Source: CAD feature listing. Evaluate the final solid. Frame: model axes, mm. A direction names the side the tool comes from. Round coordinates to 2 decimals unless told otherwise and drop trailing zeros. Loops run counter-clockwise (first coordinate to the right, second up) from the corner with the lowest first, then second, coordinate; pieces in that order, holes last. Notation, with made-up numbers: (6, 3.25) -> (10, 3.25) arc R21 ccw to (10, 42.25) -> close; hole circle Ø4 at (-6, -5.5). An arc over 180 degrees is marked (long way). Put each result on its own line as item: value. Start each with the question number.
1. Cut plane A-A (y = 0). Return the cut outline in (x, z), then the cut area to 3 significant figures.
2. Cut plane D-D (y = 7.25). Return the cut outline in (x, z).
3. Cut plane B-B (z = 1). Return the cut outline in (x, y).
4. Cut plane C-C (x = 0). Return the cut outline in (y, z), then the cut area to 3 significant figures.
5. Set-up query: faces 1 (the flat face through (-14.345, 6.755, 2.465)), 2 (the flat face through (-2, 6, 5)). Return all of +Z, -Z, +X, -X, +Y, -Y with unobstructed straight access to the full face (end or side cutting, diameter ignored); none if empty.
6. Material intervals for L1, parallel to Y at x = 0, z = 6.2; L2, parallel to Z at x = -26, y = -1.5; L3, parallel to Y at x = 0, z = 2.7, sorted ascending.
7. Draft query along X for faces 3 (the flat face through (-14.015, -6.836, 2.465)), 4 (the cylindrical face through (-6, 0, 6)), 5 (the cylindrical face through (-1.73, -7.81, 2.46)), 6 (the flat face through (0, -7, 7)). Return one class per face: pulls with the +X half, pulls with the -X half, needs draft (parallel to the pull), parting line crosses it, or undercut.
8. Contact query for flat-ended pins moving along their axis: pin 1 (3 mm diameter, centred on x = -21.5, z = 5.5, fed in from -Y); pin 2 (1.5 mm diameter, centred on x = -20.5, y = 0, fed in from -Z); pin 3 (6 mm diameter, centred on x = -21.5, y = 1.5, fed in from +Z); pin 4 (1 mm diameter, centred on x = -11.5, z = 2.5, fed in from +Y). Output: stop coordinate, or through.
```python
from build123d import *

# Parameters (mm, degrees)
SKETCH_R      = 8
PAD_DEPTH     = 5
SKETCH001_R   = 10
SKETCH001_R_2 = 6
PAD001_DEPTH  = 2


with BuildPart() as part:
    # Sketch → Pad (new body)
    with BuildSketch(Plane.XY):
        with BuildLine():
            ThreePointArc((-2.4, -9.707729), (10, 0), (-2.4, 9.707729))
            Line((-25.96, 3.883092), (-2.4, 9.707729))
            ThreePointArc((-25.96, 3.883092), (-29, 0), (-25.96, -3.883092))
            Line((-2.4, -9.707729), (-25.96, -3.883092))
        make_face()
        Circle(SKETCH_R, mode=Mode.SUBTRACT)
    extrude(amount=PAD_DEPTH)

    # Sketch001 (on Face7 of Pad) → Pad001 (join)
    with BuildSketch(Plane.XY.offset(5)):
        Circle(SKETCH001_R)
        Circle(SKETCH001_R_2, mode=Mode.SUBTRACT)
    extrude(amount=PAD001_DEPTH)


solid = part.part
```
Solution:
1. outline: (-29, 0) -> (-8, 0) -> (-8, 5) -> (-6, 5) -> (-6, 7) -> (-10, 7) -> (-10, 5) -> (-29, 5) -> close; (6, 5) -> (8, 5) -> (8, 0) -> (10, 0) -> (10, 7) -> (6, 7) -> close
1. area: 131 mm^2
2. outline: (-12.34, 0) -> (-3.38, 0) -> (-3.38, 5) -> (3.38, 5) -> (3.38, 0) -> (6.89, 0) -> (6.89, 7) -> (-6.89, 7) -> (-6.89, 5) -> (-12.34, 5) -> close
3. outline: (-25.96, -3.88) -> (-2.4, -9.71) arc R10 ccw (long way) to (-2.4, 9.71) -> (-25.96, 3.88) arc R4 ccw to start; hole circle Ø16 at (0, 0)
4. outline: (-10, 0) -> (-8, 0) -> (-8, 5) -> (-6, 5) -> (-6, 7) -> (-10, 7) -> close; (6, 5) -> (8, 5) -> (8, 0) -> (10, 0) -> (10, 7) -> (6, 7) -> close
4. area: 36.0 mm^2
5. face 1: +Z, -Z, -X, +Y
5. face 2: -Z
6. L1: y = -10 to -6, 6 to 10
6. L2: z = 0 to 5
6. L3: y = -10 to -8, 8 to 10
7. face 3: pulls with the -X half
7. face 4: undercut
7. face 5: undercut
7. face 6: needs draft
8. pin 1: stops at y = -5.34
8. pin 2: stops at z = 0
8. pin 3: stops at z = 5
8. pin 4: stops at y = 7.58
